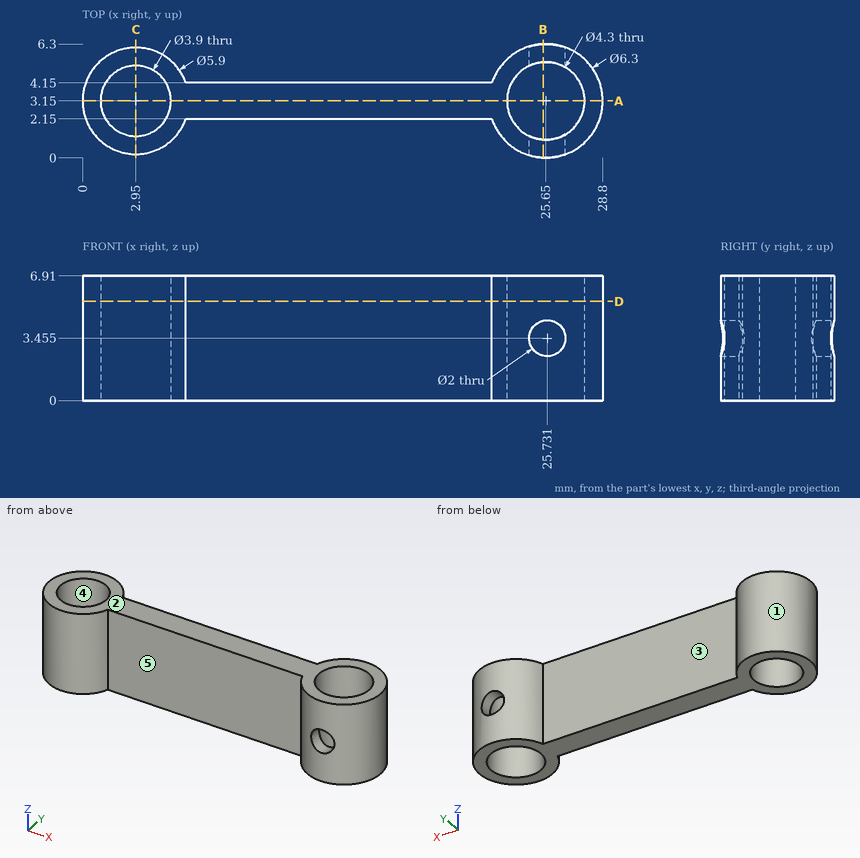
Can you work these out from the drawing? Everything is in mm from the part's minimum corner. A direction names the side the tool comes from. Give positions to 0.01 mm unless a question says otherwise; leave off trailing zeros. Loops run counter-clockwise (first coordinate to the right, second up) from the corner with the lowest first, then second, coordinate; pieces in that order, holes last. Notation, with made-up numbers: (24, 61.5) -> (37, 61.5) arc R24 cw to (37, 83.5) -> close; hole circle Ø8 at (-9.75, 34). An arc over 180 degrees is marked (long way). Return JSON: item names as keys, results as strings.
Item 1: If we section it at C-C on x = 2.95: List the corners of the cut face in (y, z) for me, plus the area to 3 significant figures.
Geometry results:
{"outline": "(0.2, 0) -> (1.2, 0) -> (1.2, 6.91) -> (0.2, 6.91) -> close; (5.1, 0) -> (6.1, 0) -> (6.1, 6.91) -> (5.1, 6.91) -> close", "area": "13.8 mm²"}
Item 2: If we section it at B-B on x = 25.5: List the corners of the cut face in (y, z) for me (1 decimal).
Geometry results:
{"outline": "(0, 0) -> (1, 0) -> (1, 2.5) -> (0, 2.5) -> close; (0, 4.4) -> (1, 4.4) -> (1, 6.9) -> (0, 6.9) -> close; (5.3, 0) -> (6.3, 0) -> (6.3, 2.5) -> (5.3, 2.5) -> close; (5.3, 4.4) -> (6.3, 4.4) -> (6.3, 6.9) -> (5.3, 6.9) -> close"}
Item 3: Which directions (+Z, -Z, +X, -X, +Y, -Y) give clear straight access to the entire face, cutting with the end or side of a thin tool? Please do the marked faces 3, 4 and 5.
Geometry results:
{"face 3": "+Z, -Z, +Y", "face 4": "+Z, -Z", "face 5": "+Z, -Z, -Y"}
Item 4: We'd pull the mould along X, two halves only. Please class the marked faces 1 and 2: +X half, -X half, draft (parallel to the pull), parting line (faces both ways), or undercut.
Geometry results:
{"face 1": "undercut", "face 2": "draft"}
Item 5: I'm going to push flat-ended pins straight in: pin 1 (3 mm diameter, centred on x = 25.73, z = 3.46, fed in from -Y); pin 2 (1 mm diameter, centred on x = 8, z = 5, fed in from -Y); pin 3 (2 mm diameter, centred on y = 0.5, z = 5, fed in from -X) (1 decimal); pin 4 (1.5 mm diameter, centred on y = 1.5, z = 6, fed in from +X). Where does each tip first touch, or does it pass through?
Geometry results:
{"pin 1": "stops at y = 0", "pin 2": "stops at y = 2.15", "pin 3": "stops at x = 0.5", "pin 4": "stops at x = 28.67"}
Item 6: I need wall thicknesses on L1, parallel to X at y = 3, z = 2.5 (1 decimal); L2, parallel to X at y = 4.5, z = 5.5 (1 decimal); L3, parallel to Y at x = 2.95, z = 2.5. Which ranges of each line are inside material? Lowest first, please. Write a range as from..to.
Geometry results:
{"L1": "x = 0..1, 4.9..23.5, 27.8..28.8", "L2": "x = 0.3..1.5, 4.4..5.6, 22.8..24, 27.3..28.5", "L3": "y = 0.2..1.2, 5.1..6.1"}
Item 7: If we section it at A-A on y = 3.15: List the corners of the cut face in (x, z) for me.
Geometry results:
{"outline": "(0, 0) -> (1, 0) -> (1, 6.91) -> (0, 6.91) -> close; (4.9, 0) -> (23.5, 0) -> (23.5, 6.91) -> (4.9, 6.91) -> close; (27.8, 0) -> (28.8, 0) -> (28.8, 6.91) -> (27.8, 6.91) -> close"}
Item 8: If we section it at D-D on z = 5.5: Count the separate pieces of the cut face and the enclosed holes in it.
Geometry results:
{"separate pieces": "1", "enclosed holes": "2"}
